Here's the drawing with two shaded views (mm, measured from the low corner). I have some questions. Give positions to 0.01 mm unless a question says otherwise; leave off trailing zeros. Order: outer loops, then holes, each group sorted by start corner. A loop starts at its lowest first (then second) coordinate and runs counter-clockwise, first axis right, second up. Notation, with made-up numbers: (25, 77.25) - (69, 77.25) arc R14 ccw to (69, 85.25) - close; hole circle Ø4 at (62.25, 66). An arc over 180 degrees is marked (long way). Use one line per item in the form item = value. Start each with the question number.
1) Suppose I cut it at A-A, the plane x = 10. Write out the boundary of the cut face in (y, z).
2) For pin 1 (5.5 mm diameter, centred on x = 26, z = 96, fed in from -Y); pin 2 (6 mm diameter, centred on x = 13.5, z = 48.5, fed in from +Y); pin 3 (2 mm diameter, centred on x = 31.5, y = 26.5, fed in from +Z), each with a flat end and sliding along its axis, tell me the tip position at first contact or that it passes through.
3) Suppose I cut it at C-C, the plane z = 124. Write out the boundary of the cut face in (x, y), and give its area (3 significant figures).
4) Please list where these lines run through material, in increasing order: probe 1 along Z at (x, y) = (26, 14.4); probe 2 along Y at (x, z) = (18, 3.25); probe 3 along Y at (x, z) = (26.5, 141).
5) Suppose I cut it at B-B, the plane y = 5.5. Write out the boundary of the cut face in (x, z).
6) We'd pull the mould along Z, two halves only. Please class the marked faces 1 and 2: released by +Z, released by -Z, zero draft, split by the parting line, or undercut.
7) Suppose I cut it at D-D, the plane z = 37. Write out the boundary of the cut face in (x, y), and give its area (3 significant figures).
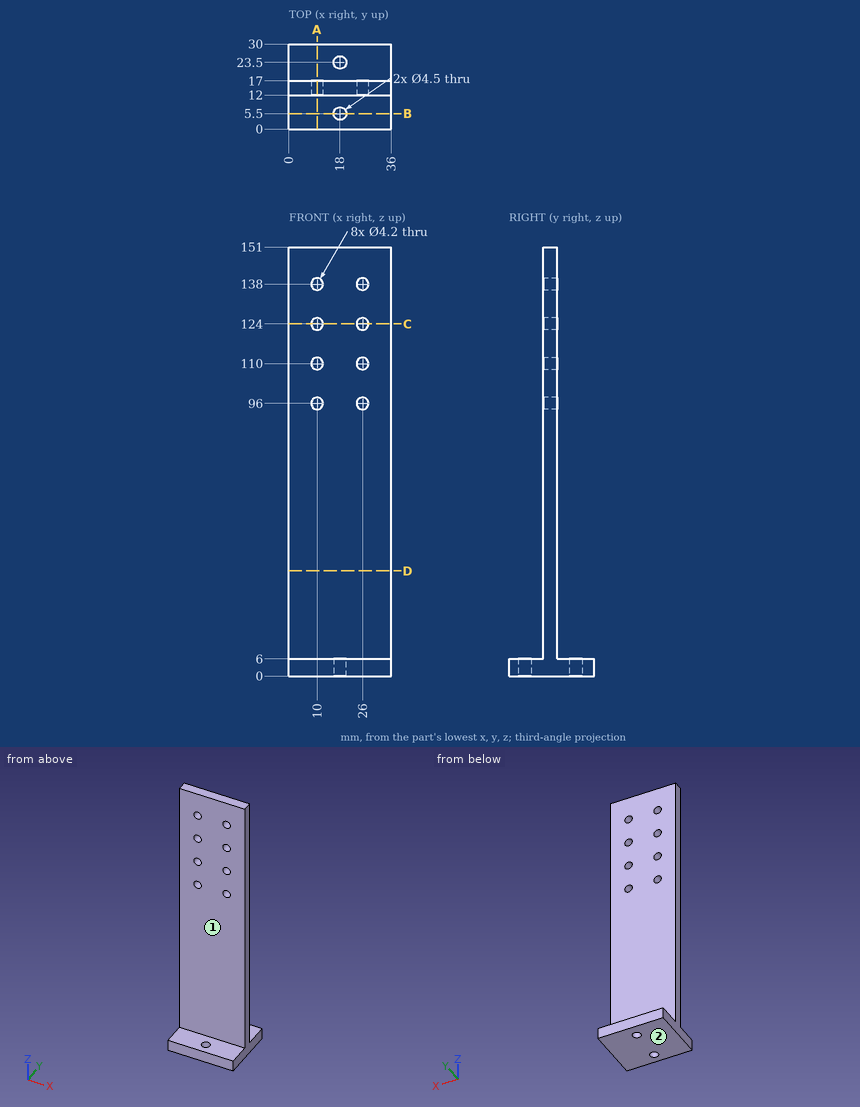
Result sheet:
q1.outline = (0, 0) - (30, 0) - (30, 6) - (17, 6) - (17, 93.9) - (12, 93.9) - (12, 6) - (0, 6) - close; (12, 98.1) - (17, 98.1) - (17, 107.9) - (12, 107.9) - close; (12, 112.1) - (17, 112.1) - (17, 121.9) - (12, 121.9) - close; (12, 126.1) - (17, 126.1) - (17, 135.9) - (12, 135.9) - close; (12, 140.1) - (17, 140.1) - (17, 151) - (12, 151) - close
q2.pin_1 = 12
q2.pin_2 = 17
q2.pin_3 = 6
q3.outline = (0, 12) - (7.9, 12) - (7.9, 17) - (0, 17) - close; (12.1, 12) - (23.9, 12) - (23.9, 17) - (12.1, 17) - close; (28.1, 12) - (36, 12) - (36, 17) - (28.1, 17) - close
q3.area = 138 mm²
q4.probe_1 = 0 to 93.9, 98.1 to 107.9, 112.1 to 121.9, 126.1 to 135.9, 140.1 to 151
q4.probe_2 = 0 to 3.25, 7.75 to 21.25, 25.75 to 30
q4.probe_3 = 12 to 17
q5.outline = (0, 0) - (15.75, 0) - (15.75, 6) - (0, 6) - close; (20.25, 0) - (36, 0) - (36, 6) - (20.25, 6) - close
q6.face_1 = zero draft
q6.face_2 = released by -Z
q7.outline = (0, 12) - (36, 12) - (36, 17) - (0, 17) - close
q7.area = 180 mm²
